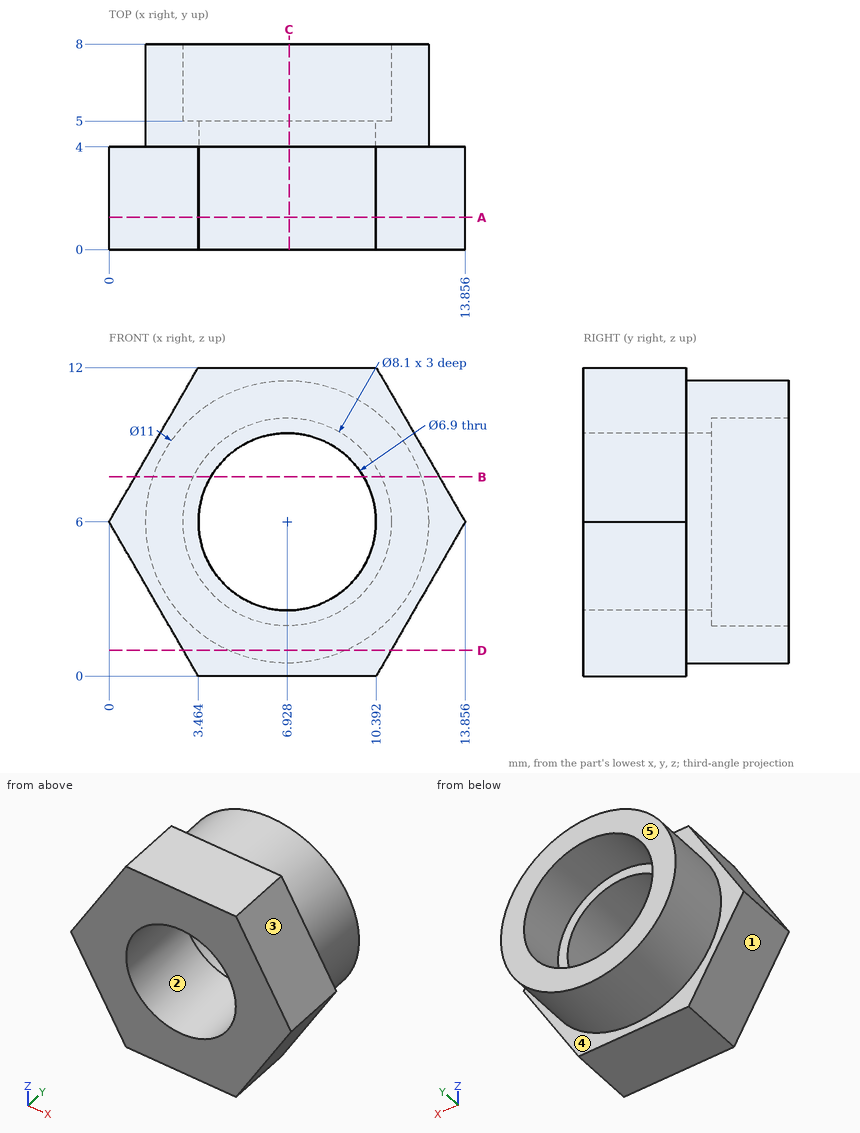
Can you work these out from the drawing? Everything is in mm from the part's minimum corner. A direction names the side the tool comes from. Round coordinates to 2 decimals unless told otherwise and drop trailing zeros. Loops run counter-clockwise (first coordinate to the right, second up) from the corner with the lowest first, then second, coordinate; pieces in that order, holes last. Notation, with made-up numbers: M 86,87 L 115,87 A18 ccw 115,92 Z; hole C -16,3.5 d10. An arc over 180 degrees is marked long. Write item = value, one per line.
1. I want a section at A-A, the plane y = 1.25. Write out the boundary of the cut face in (x, z).
Results below:
outline = M 0,6 L 3.46,0 L 10.39,0 L 13.86,6 L 10.39,12 L 3.46,12 Z; hole C 6.93,6 d6.9
2. Which directions (+Z, -Z, +X, -X, +Y, -Y) give clear straight access to the entire face, cutting with the end or side of a thin tool? Please do the marked faces 4 and 5.
Results below:
face_4 = +Y
face_5 = +Z, -Z, +X, -X, +Y
3. I need wall thicknesses on probe 1 along Z at (x, y) = (8.75, 3); probe 2 along X at (y, z) = (3.75, 4) (1 decimal); probe 3 along X at (y, z) = (2.5, 3) (1 decimal). Which ranges of each line are inside material? Lowest first, please.
Results below:
probe_1 = 0 to 3.07, 8.93 to 12
probe_2 = 1.2 to 4.1, 9.7 to 12.7
probe_3 = 1.7 to 5.2, 8.6 to 12.1
4. I want a section at B-B, the plane z = 7.75. Write out the boundary of the cut face in (x, y) (1 decimal), and give its area (3 significant figures).
Results below:
outline = M 1,0 L 4,0 L 4,5 L 3.3,5 L 3.3,8 L 1.7,8 L 1.7,4 L 1,4 Z; M 9.9,0 L 12.8,0 L 12.8,4 L 12.1,4 L 12.1,8 L 10.6,8 L 10.6,5 L 9.9,5 Z
area = 37.4 mm²
5. Will these pins go through, and if not, where does the flat tip stop? P1, Ø2, axis at y = 1.5, z = 3.5, coming from the +X side; P2, Ø1.5, axis at x = 8.5, y = 6.5, coming from the +Z side.
Results below:
P1 = 12.99
P2 = 11.44
6. Thinking about a two-plate mould opening in Z: for the marked faces 1, 2 and 3, which applies, +Z half, -Z half, draft (parallel to the pull), parting line (faces both ways), or undercut?
Results below:
face_1 = -Z half
face_2 = undercut
face_3 = +Z half
7. I want a section at C-C, the plane x = 7. Write out the boundary of the cut face in (y, z).
Results below:
outline = M 0,0 L 4,0 L 4,0.5 L 8,0.5 L 8,1.95 L 5,1.95 L 5,2.55 L 0,2.55 Z; M 0,9.45 L 5,9.45 L 5,10.05 L 8,10.05 L 8,11.5 L 4,11.5 L 4,12 L 0,12 Z
8. I want a section at D-D, the plane z = 1. Write out the boundary of the cut face in (x, y).
Results below:
outline = M 2.89,0 L 10.97,0 L 10.97,4 L 9.22,4 L 9.22,8 L 4.64,8 L 4.64,4 L 2.89,4 Z
